Read the model definition and answer for the solid it produces. Units are mm, in the model's axes. A direction names the side the tool comes from. Coordinates: 2 decimals unless noted, no trailing zeros. Loops run counter-clockwise (first coordinate to the right, second up) from the corner with the lowest first, then second, coordinate; pieces in that order, holes last. Notation, with made-up numbers: (-9.5, -29) -> (20.5, -29) arc R5 cw to (20.5, -25) -> close; hole circle Ø3 at (88, 66.25). An arc over 180 degrees is marked (long way). Answer as CSV lines item,"result".
```python
from build123d import *

# Parameters (mm, degrees)
F0_R     = 4
F0_R_2   = 3
F1_DEPTH = 7
F2_R     = 3
F3_DEPTH = 1
F4_SIZE  = 1
F5_R     = 0.25


with BuildPart() as f1:
    # F0 (on Top) → F1 (new body)
    with BuildSketch(Plane.XY):
        Circle(F0_R)
        Circle(F0_R_2, mode=Mode.SUBTRACT)
    extrude(amount=F1_DEPTH)

    # F2 (on face) → F3 (join)
    with BuildSketch(Plane.XY.offset(7)):
        with BuildLine():
            ThreePointArc((6.204836823, -0.75), (6.2386989887, -0.3756792889), (6.25, 0))
            ThreePointArc((6.25, 0), (6.2386989887, 0.3756792889), (6.204836823, 0.75))
            Line((6.204836823, 0.75), (5.5, 0.75))
            Line((5.5, 0.75), (5.5, -0.75))
            Line((5.5, -0.75), (6.204836823, -0.75))
        make_face()
        with BuildLine():
            ThreePointArc((6.204836823, 0.75), (6.2386989887, 0.3756792889), (6.25, 0))
            ThreePointArc((6.25, 0), (6.2386989887, -0.3756792889), (6.204836823, -0.75))
            Line((6.204836823, -0.75), (7, -0.75))
            Line((7, -0.75), (7, 0.75))
            Line((7, 0.75), (6.204836823, 0.75))
        make_face()
        with BuildLine():
            Line((5.5, 0.75), (6.204836823, 0.75))
            ThreePointArc((6.204836823, 0.75), (4.4194173824, 4.4194173824), (0.75, 6.204836823))
            Line((0.75, 6.204836823), (0.75, 5.5))
            Line((0.75, 5.5), (-0.75, 5.5))
            Line((-0.75, 5.5), (-0.75, 6.204836823))
            ThreePointArc((-0.75, 6.204836823), (-4.4194173824, 4.4194173824), (-6.204836823, 0.75))
            Line((-6.204836823, 0.75), (-5.5, 0.75))
            Line((-5.5, 0.75), (-5.5, -0.75))
            Line((-5.5, -0.75), (-6.204836823, -0.75))
            ThreePointArc((-6.204836823, -0.75), (-4.4194173824, -4.4194173824), (-0.75, -6.204836823))
            Line((-0.75, -6.204836823), (-0.75, -5.5))
            Line((-0.75, -5.5), (0.75, -5.5))
            Line((0.75, -5.5), (0.75, -6.204836823))
            ThreePointArc((0.75, -6.204836823), (4.4194173824, -4.4194173824), (6.204836823, -0.75))
            Line((6.204836823, -0.75), (5.5, -0.75))
            Line((5.5, -0.75), (5.5, 0.75))
        make_face()
        Circle(F2_R, mode=Mode.SUBTRACT)
        with BuildLine():
            Line((0.75, 5.5), (0.75, 6.204836823))
            ThreePointArc((0.75, 6.204836823), (0, 6.25), (-0.75, 6.204836823))
            Line((-0.75, 6.204836823), (-0.75, 5.5))
            Line((-0.75, 5.5), (0.75, 5.5))
        make_face()
        with BuildLine():
            ThreePointArc((-0.75, 6.204836823), (0, 6.25), (0.75, 6.204836823))
            Line((0.75, 6.204836823), (0.75, 7))
            Line((0.75, 7), (-0.75, 7))
            Line((-0.75, 7), (-0.75, 6.204836823))
        make_face()
        with BuildLine():
            Line((0.75, -7), (0.75, -6.204836823))
            ThreePointArc((0.75, -6.204836823), (0, -6.25), (-0.75, -6.204836823))
            Line((-0.75, -6.204836823), (-0.75, -7))
            Line((-0.75, -7), (0.75, -7))
        make_face()
        with BuildLine():
            ThreePointArc((-0.75, -6.204836823), (0, -6.25), (0.75, -6.204836823))
            Line((0.75, -6.204836823), (0.75, -5.5))
            Line((0.75, -5.5), (-0.75, -5.5))
            Line((-0.75, -5.5), (-0.75, -6.204836823))
        make_face()
        with BuildLine():
            Line((-5.5, 0.75), (-6.204836823, 0.75))
            ThreePointArc((-6.204836823, 0.75), (-6.25, 0), (-6.204836823, -0.75))
            Line((-6.204836823, -0.75), (-5.5, -0.75))
            Line((-5.5, -0.75), (-5.5, 0.75))
        make_face()
        with BuildLine():
            ThreePointArc((-6.204836823, -0.75), (-6.25, 0), (-6.204836823, 0.75))
            Line((-6.204836823, 0.75), (-7, 0.75))
            Line((-7, 0.75), (-7, -0.75))
            Line((-7, -0.75), (-6.204836823, -0.75))
        make_face()
    extrude(amount=F3_DEPTH)

    # F4
    f4_edges = [f1.edges().sort_by_distance(p)[0] for p in [
        (-3, 0, 8),
        (-4, 0, 7),
    ]]
    chamfer(f4_edges, length=F4_SIZE)

    # F5
    f5_edges = [f1.edges().sort_by_distance(p)[0] for p in [
        (-7, -0.75, 7.5),
        (-7, 0.75, 7.5),
        (-0.75, -7, 7.5),
        (0.75, -7, 7.5),
        (7, -0.75, 7.5),
        (7, 0.75, 7.5),
        (0.75, 7, 7.5),
        (-0.75, 7, 7.5),
        (-4, 0, 8),
        (6.602418, -0.75, 8),
        (7, 0, 8),
        (6.602418, 0.75, 8),
        (4.419417, 4.419417, 8),
        (0.75, 6.602418, 8),
        (0, 7, 8),
        (-0.75, 6.602418, 8),
        (-4.419417, 4.419417, 8),
        (-6.602418, 0.75, 8),
        (-7, 0, 8),
        (-6.602418, -0.75, 8),
        (-4.419417, -4.419417, 8),
        (-0.75, -6.602418, 8),
        (0, -7, 8),
        (0.75, -6.602418, 8),
        (4.419417, -4.419417, 8),
    ]]
    fillet(f5_edges, radius=F5_R)


solid = f1.part
```
Q1. A cutting plane is placed at A-A, the plane y = 0. Write down the section's boundary in (x, z), and give its area (3 significant figures).
Results:
outline,"(-7, 7) -> (-5, 7) -> (-4, 6) -> (-4, 0) -> (-3, 0) -> (-3, 7) -> (-3.93, 7.93) arc R0.25 ccw to (-4.1, 8) -> (-6.75, 8) arc R0.25 ccw to (-7, 7.75) -> close; (3, 0) -> (4, 0) -> (4, 6) -> (5, 7) -> (7, 7) -> (7, 7.75) arc R0.25 ccw to (6.75, 8) -> (4.1, 8) arc R0.25 ccw to (3.93, 7.93) -> (3, 7) -> close"
area,"22.0 mm²"
Q2. Find the intervals of material crossed by probe 1 along Y at (x, z) = (0, 4.5); probe 2 along Z at (x, y) = (2, 5.5); probe 3 along X at (y, z) = (-1.75, 3.5), in increasing order. Write a range as [from, to].
Results:
probe 1,"y = [-4, -3], [3, 4]"
probe 2,"z = [7, 8]"
probe 3,"x = [-3.6, -2.44], [2.44, 3.6]"
Q3. A cutting plane is placed at D-D, the plane z = 5. Write down the section's boundary in (x, y).
Results:
outline,"circle Ø8 at (0, 0); hole circle Ø6 at (0, 0)"
Q4. A cutting plane is placed at C-C, the plane z = 7.5. Write down the section's boundary in (x, y), and give its area (3 significant figures).
Results:
outline,"(-7, -0.5) arc R0.25 ccw to (-6.75, -0.75) -> (-6.2, -0.75) arc R6.25 ccw to (-0.75, -6.2) -> (-0.75, -6.75) arc R0.25 ccw to (-0.5, -7) -> (0.5, -7) arc R0.25 ccw to (0.75, -6.75) -> (0.75, -6.2) arc R6.25 ccw to (6.2, -0.75) -> (6.75, -0.75) arc R0.25 ccw to (7, -0.5) -> (7, 0.5) arc R0.25 ccw to (6.75, 0.75) -> (6.2, 0.75) arc R6.25 ccw to (0.75, 6.2) -> (0.75, 6.75) arc R0.25 ccw to (0.5, 7) -> (-0.5, 7) arc R0.25 ccw to (-0.75, 6.75) -> (-0.75, 6.2) arc R6.25 ccw to (-6.2, 0.75) -> (-6.75, 0.75) arc R0.25 ccw to (-7, 0.5) -> close; hole circle Ø7 at (0, 0)"
area,"88.7 mm²"
Q5. For faces 1 (the face through (-0.867, -3.905, 2.958)), 2 (the face through (-4.38, 4.46, 7.37)), determine the directions among +Z, -Z, +X, -X, +Y, -Y from which every point of the face is accessible in a straight line to the end or side of a thin tool.
Results:
face 1,"-Z"
face 2,"+Z, -Z, -X, +Y"
Q6. Given pin 1 Ø3 at (y, z) = (-4, 2.5) entering from -X; pin 2 Ø4 at (x, z) = (-2.5, 4) entering from +Y; pin 3 Ø2 at (x, y) = (4, -5) entering from -Z, each flat-ended and moving along its own axis, determine where each tip first touches the part or whether it passes through.
Results:
pin 1,"stops at x = -3.12"
pin 2,"stops at y = 3.97"
pin 3,"stops at z = 7"
Q7. For a pull along X with two mould halves and no side action, classify faces 3 (the face through (5, 2, 7)), 4 (the face through (-3, 0, 3)), 5 (the face through (4.38, -4.46, 7.37)) as pulls with the +X half, pulls with the -X half, needs draft (parallel to the pull), parting line crosses it, or undercut.
Results:
face 3,"needs draft"
face 4,"undercut"
face 5,"pulls with the +X half"
